Model file for the job. Use its own axes, mm. Face numbers are marked on the shaded views. Coordinates: 2 decimals unless noted, no trailing zeros. Write each loop counter-clockwise with the first axis right and the second up, starting at its lowest first coordinate (ties: lowest second). Pieces come first, ordered by that corner, then holes. Notation, with made-up numbers: M 20.25,67 L 32.25,67 A17 cw 32.25,90 Z; hole C 82,36 d6. An arc over 180 degrees is marked long. Answer in a Markdown table with one row per item. Add a question column.
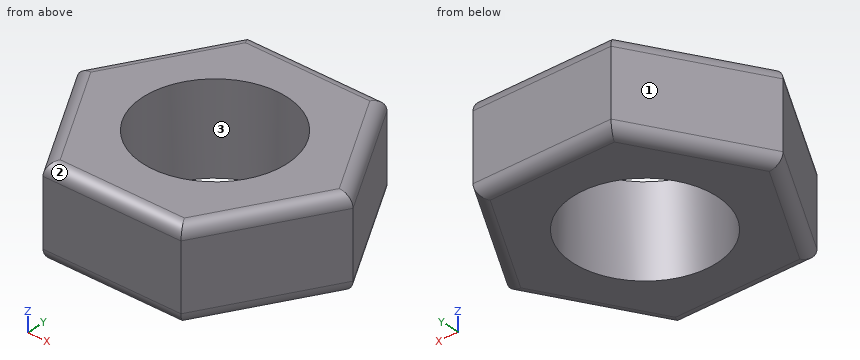
```python
from build123d import *

# Parameters (mm, degrees)
EXTRUDE_3_DEPTH     = 7.5
FILLET_3_R          = 1
SKETCH_4_R          = 6
CUT_EXTRUDE_1_DEPTH = 18.017148214


with BuildPart() as part:
    # 草图1 → 凸台-拉伸3 (new body)
    with BuildSketch(Plane.XY):
        Polygon((5.773502692, -10), (11.547005384, 0), (5.773502692, 10), (-5.773502692, 10), (-11.547005384, 0), (-5.773502692, -10), align=None)
    extrude(amount=EXTRUDE_3_DEPTH)

    # 圆角3
    fillet_3_edges = [part.edges().sort_by_distance(p)[0] for p in [
        (8.660254038, 5, 7.5),
        (0, 10, 7.5),
        (-8.660254038, 5, 7.5),
        (-8.660254038, -5, 7.5),
        (0, -10, 7.5),
        (-8.660254038, -5, 0),
        (-8.660254038, 5, 0),
        (0, 10, 0),
        (8.660254038, -5, 7.5),
        (8.660254038, 5, 0),
        (8.660254038, -5, 0),
        (0, -10, 0),
    ]]
    fillet(fillet_3_edges, radius=FILLET_3_R)

    # 草图4 → 切除-拉伸1 (cut, through all)
    with BuildSketch(Plane.XY.offset(7.5)):
        Circle(SKETCH_4_R)
    extrude(amount=-CUT_EXTRUDE_1_DEPTH, mode=Mode.SUBTRACT)


solid = part.part
```
1) Drill centre lines: probe 1 along Y at (x, z) = (0, 4.25); probe 2 along X at (y, z) = (2.75, 3.75); probe 3 along X at (y, z) = (-4.25, 3.5). Where is each one in solid material? Low to high.
2) Flat gauge pin, fed straight in: pin 1 Ø2 at (y, z) = (7, 6) entering from +X. Where does the tip first touch, or does it go through?
3) Two-plate mould, pull along Y, no slides. Class the marked faces 1, 2 and 3: released by +Y, released by -Y, zero draft, split by the parting line, or undercut.
4) Slice it at C-C (x = -2.75). Give the cut face in (y, z), then the cut area to 3 significant figures.
5) Slice it at A-A (x = 0). Give the cut face in (y, z), then the cut area to 3 significant figures.
6) Slice it at B-B (z = 4.75). Give the cut face in (x, y).
Ans:
| question | item | result |
|---|---|---|
| 1 | probe 1 | y = -10 to -6, 6 to 10 |
| 1 | probe 2 | x = -9.96 to -5.33, 5.33 to 9.96 |
| 1 | probe 3 | x = -9.09 to -4.24, 4.24 to 9.09 |
| 2 | pin 1 | stops at x = 8.08 |
| 3 | face 1 | released by +Y |
| 3 | face 2 | released by -Y |
| 3 | face 3 | undercut |
| 4 | outline | M -10,1 A1 ccw -9,0 L -5.33,0 L -5.33,7.5 L -9,7.5 A1 ccw -10,6.5 Z; M 5.33,0 L 9,0 A1 ccw 10,1 L 10,6.5 A1 ccw 9,7.5 L 5.33,7.5 Z |
| 4 | area | 69.2 mm2 |
| 5 | outline | M -10,1 A1 ccw -9,0 L -6,0 L -6,7.5 L -9,7.5 A1 ccw -10,6.5 Z; M 6,0 L 9,0 A1 ccw 10,1 L 10,6.5 A1 ccw 9,7.5 L 6,7.5 Z |
| 5 | area | 59.1 mm2 |
| 6 | outline | M -11.55,0 L -5.77,-10 L 5.77,-10 L 11.55,0 L 5.77,10 L -5.77,10 Z; hole C 0,0 d12 |
